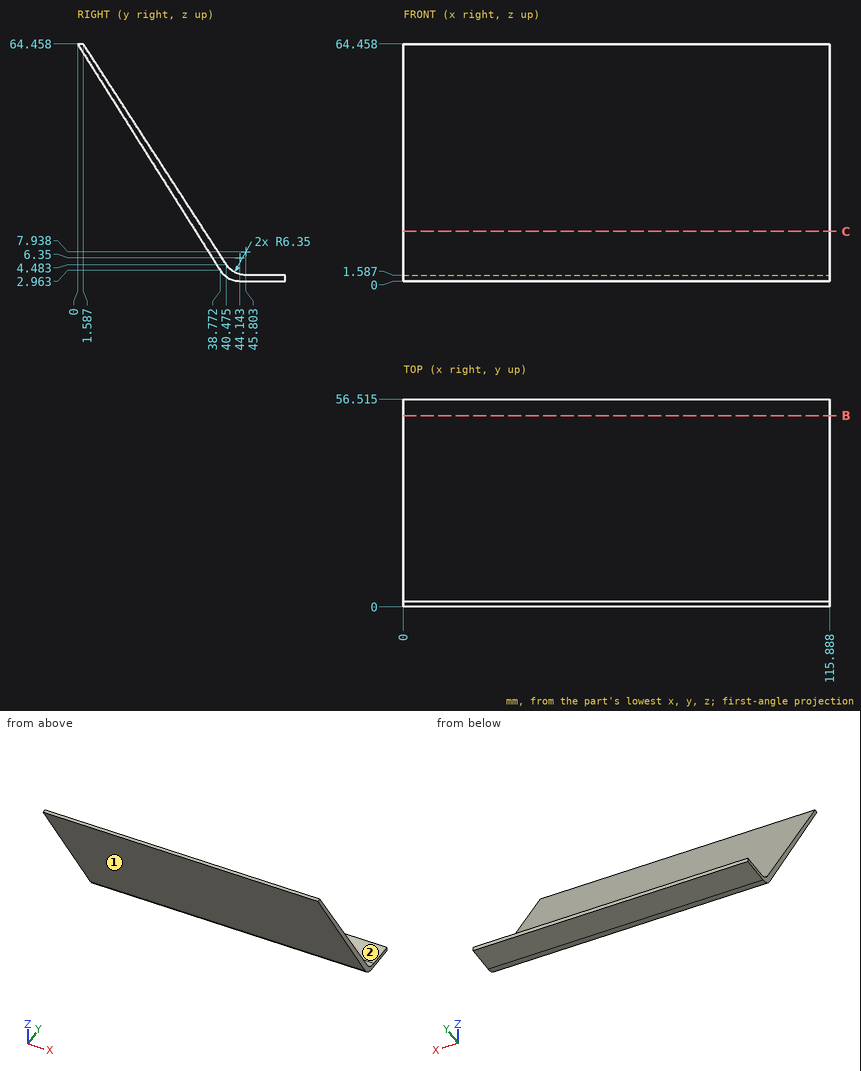
Drawing for the job (mm, zero at the part's lowest x, y, z). A direction names the side the tool comes from. Coordinates: 2 decimals unless noted, no trailing zeros. Order: outer loops, then holes, each group sorted by start corner. A loop starts at its lowest first (then second) coordinate and runs counter-clockwise, first axis right, second up. Notation, with made-up numbers: (9.25, 18) - (13.25, 18) arc R32 ccw to (13.25, 56) - close; hole circle Ø3 at (22, 10.5). An arc over 180 degrees is marked (long way). Use a Markdown table: item, result. Add a question column.
(1) Saw through at C-C (z = 13.5). Give the cut face in (x, y), then the cut area to 3 significant figures.
(2) Saw through at B-B (y = 52). Give the cut face in (x, z), then the cut area to 3 significant figures.
(3) Which spindle directions (+Z, -Z, +X, -X, +Y, -Y) get a long thin tool onto all of the face, cutting with end or side? Do the marked faces 1 and 2. Say none if no direction does.
(4) Flat gauge pins, fed straight in: pin 1 (1 mm diameter, centred on x = 82.5, y = 7, fed in from -Z) (1 decimal); pin 2 (3 mm diameter, centred on x = 66.5, y = 16.5, fed in from +Z) (1 decimal); pin 3 (4 mm diameter, centred on x = 56.5, z = 9, fed in from +Y). Where does each tip first touch, or does it go through?
(5) Drill centre lines: line 1 along Z through (x, y) = (42.5, 51); line 2 along Y through (x, z) = (67, 6) (1 decimal); line 3 along Z through (x, y) = (62, 9) (1 decimal). Where is each one in solid material? Low to high. Write a range as [from, to].
Solved:
| question | item | result |
|---|---|---|
| 1 | outline | (0, 32.13) - (115.89, 32.13) - (115.89, 34.63) - (0, 34.63) - close |
| 1 | area | 290 mm² |
| 2 | outline | (0, 0) - (115.89, 0) - (115.89, 1.59) - (0, 1.59) - close |
| 2 | area | 184 mm² |
| 3 | face 1 | -Z, +X, -X, -Y |
| 3 | face 2 | +Z, +X, -X, +Y |
| 4 | pin 1 | stops at z = 52.6 |
| 4 | pin 2 | stops at z = 43.8 |
| 4 | pin 3 | stops at y = 38.84 |
| 5 | line 1 | z = [0, 1.59] |
| 5 | line 2 | y = [36.9, 39.5] |
| 5 | line 3 | z = [50.2, 53] |
